The model under review builds one solid part; all positions refer to its coordinate system, in mm. A direction names the side the tool comes from. Give positions to 0.01 mm unless a question says otherwise; leave off trailing zeros. Loops run counter-clockwise (first coordinate to the right, second up) from the corner with the lowest first, then second, coordinate; pieces in that order, holes last. Notation, with made-up numbers: M 87,-19.5 L 95,-19.5 A32 ccw 95,17.5 Z; hole C 66,61.25 d5. An arc over 180 degrees is marked long. Write item = value, one per line. Start each with the question number.
1. Draft analysis for pull direction X (two halves, no side actions). For faces 6 (the face through (6, 38.1, -24)), 7 (the face through (-19.89, 22, 18.24)), 8 (the face through (6, 0, -24)), 9 (the face through (13, 2.54, -24)), state which applies: pulls with the +X half, pulls with the -X half, needs draft (parallel to the pull), parting line crosses it, or undercut.
2. We need section C-C on y = -91.5. Give the boundary of the cut face in (x, z) (1 decimal), then the cut area to 3 significant figures.
3. Wall thickness on line 1 along Y through (x, z) = (-46.5, -11); line 2 along Z through (x, y) = (0, 1); line 3 along Z through (x, y) = (5, -86.5): over which ranges is each line inside the solid? List them lowest first. Write a range as from..to.
4. We need section D-D on z = -38. Give the boundary of the cut face in (x, y).
5. For faces 1 (the face through (-19.89, -48.84, 18.24)), 2 (the face through (22, -101.6, -22)), 3 (the face through (22, 6.35, -22)), 4 (the face through (5.875, 3.184, -26.456)), 5 (the face through (-13.2, 19.32, 20.71)), list the 3-axis set-ups (+Z, -Z, +X, -X, +Y, -Y) from which the entire face can be reached by the end or side of a thin tool; tool diameter is ignored.
6. We need section A-A on x = 0. Count the separate pieces of the cut face and the enclosed holes in it, then the cut area to 3 significant figures.
7. For pin 1 (4 mm diameter, centred on x = 24, y = 15, fed in from -Z); pin 2 (12 mm diameter, centred on y = 22.5, z = 24.5, fed in from +X); pin 3 (12 mm diameter, centred on x = 9.5, y = -54.5, fed in from +Z), all flat-tipped, find the tip position at first contact; note any pin that passes through.
from build123d import *

# Parameters (mm, degrees)
F0_R     = 26.9875
F1_DEPTH = 38.1
F0_R_2   = 50.8
F2_DEPTH = 6.35
F3_DEPTH = 101.6
F4_R     = 24.5602140896
F5_DEPTH = 127
F6_SIZE2 = 2.54
F6_SIZE  = 2.54
F7_T     = -2.54


# Not quite as in the source:
# - a feature names something its author has since deleted; it is built from what else it names


with BuildPart() as f1:
    # F0 (on Front) → F1 (new body)
    with BuildSketch(Plane.XZ):
        Circle(F0_R)
    extrude(amount=-F1_DEPTH)

    # F0 (on Front) → F2 (join)
    with BuildSketch(Plane.XZ):
        Circle(F0_R_2)
        Circle(F0_R, mode=Mode.SUBTRACT)
    extrude(amount=-F2_DEPTH)

    # F0 (on Front) → F3 (join)
    with BuildSketch(Plane.XZ):
        Circle(F0_R_2)
        Circle(F0_R, mode=Mode.SUBTRACT)
    extrude(amount=F3_DEPTH)

    # F4 (on face) → F5 (cut)
    with BuildSketch(Plane(origin=(0, 38.1, 0), x_dir=(-1, 0, 0), z_dir=(0, 1, 0))):
        Circle(F4_R)
    extrude(amount=-F5_DEPTH, mode=Mode.SUBTRACT)

    # F6
    f6_edges = [f1.edges().sort_by_distance(p)[0] for p in [
        (-26.9875, -101.6, 0),
    ]]
    chamfer(f6_edges, length=F6_SIZE, length2=F6_SIZE2)

    # F7 (hollow: no face is removed)
    offset(amount=F7_T, kind=Kind.INTERSECTION, mode=Mode.SUBTRACT)


solid = f1.part
Final values:
q1.face_6 = needs draft
q1.face_7 = parting line crosses it
q1.face_8 = undercut
q1.face_9 = undercut
q2.outline = C 0,0 d101.6; C 0,0 d59.1; hole C 0,0 d96.5; hole C 0,0 d54
q2.area = 1,240 mm²
q3.line_1 = -101.6..-99.06, 3.81..6.35
q3.line_2 = -50.8..-48.26, -29.53..-24.56, 24.56..29.53, 48.26..50.8
q3.line_3 = -50.55..-48, -29.1..-26.52, 26.52..29.1, 48..50.55
q4.outline = M -33.71,-101.6 L 33.71,-101.6 L 33.71,6.35 L -33.71,6.35 Z; hole M -29.75,-99.06 L 29.75,-99.06 L 29.75,3.81 L -29.75,3.81 Z
q5.face_1 = -Y
q5.face_2 = +Z, -Z, +X, -X, -Y
q5.face_3 = +Y
q5.face_4 = none
q5.face_5 = +Y, -Y
q6.separate_pieces = 2
q6.enclosed_holes = 2
q6.area = 1,460 mm²
q7.pin_1 = -15.63
q7.pin_2 = 19.65
q7.pin_3 = 50.68
